```python
from build123d import *

# Parameters (mm, degrees)
SKETCH1_W                   = 31.9
SKETCH1_H                   = 17.8
SKETCH1_W_2                 = 22.5
SKETCH1_H_2                 = 11.8
BOSS_EXTRUDE1_DEPTH         = 8
BOSS_EXTRUDE2_DEPTH         = 16
SKETCH5_W                   = 14.05
SKETCH5_H                   = 12
SKETCH5_W_2                 = 15.95
SKETCH5_H_2                 = 8
BOSS_EXTRUDE3_DEPTH         = 3
CUT_EXTRUDE2_DEPTH          = 3
CUT_EXTRUDE3_DEPTH          = 43.272216091
BOSS_EXTRUDE4_START         = -8
BOSS_EXTRUDE4_DEPTH         = 8
CUT_EXTRUDE4_DEPTH          = 43.128612605
IZIM1_W                     = 73.483837375
IZIM1_H                     = 17.110844689
IZIM1_R                     = 4
Y_KSEKLIK_EKSTR_ZYON1_DEPTH = 30


with BuildPart() as part:
    # Sketch1 → Boss-Extrude1 (new body)
    with BuildSketch(Plane(origin=(0, 0, 0), x_dir=(1, 0, 0), z_dir=(0, 1, 0))):
        Rectangle(SKETCH1_W, SKETCH1_H)
        Rectangle(SKETCH1_W_2, SKETCH1_H_2, mode=Mode.SUBTRACT)
    extrude(amount=BOSS_EXTRUDE1_DEPTH)

    # Sketch3 → Boss-Extrude2 (add)
    with BuildSketch(Plane.XZ):
        with BuildLine():
            ThreePointArc((28.95, -7.4), (23.95, -12.4), (18.95, -7.4))
            Line((18.95, -7.4), (18.95, 18.9))
            Line((18.95, 18.9), (15.95, 18.9))
            Line((15.95, 18.9), (15.95, -8.9))
            ThreePointArc((15.95, -8.9), (24.70323224, -15.504482784), (32.089410298, -7.4))
            Line((32.089410298, -7.4), (32.089410298, 18.9))
            Line((32.089410298, 18.9), (28.95, 18.9))
            Line((28.95, 18.9), (28.95, -7.4))
        make_face()
    extrude(amount=-BOSS_EXTRUDE2_DEPTH)

    # Sketch5 → Boss-Extrude3 (add)
    with BuildSketch(Plane(origin=(0, 0, -8.9), x_dir=(-1, 0, 0), z_dir=(0, 0, -1))):
        with Locations((-7.025, 14)):
            Rectangle(SKETCH5_W, SKETCH5_H)
        with Locations((7.975, 14)):
            Rectangle(SKETCH5_W_2, SKETCH5_H)
        with Locations((7.975, 4)):
            Rectangle(SKETCH5_W_2, SKETCH5_H_2)
        with Locations((-7.025, 4)):
            Rectangle(SKETCH5_W, SKETCH5_H_2)
    extrude(amount=BOSS_EXTRUDE3_DEPTH)

    # Sketch6 → Cut-Extrude2 (cut)
    with BuildSketch(Plane.XY.offset(-8.9)):
        with BuildLine():
            Line((-11.95, 18), (10.05, 18))
            ThreePointArc((10.05, 18), (11.05, 17), (10.05, 16))
            Line((10.05, 16), (-11.95, 16))
            ThreePointArc((-11.95, 16), (-12.95, 17), (-11.95, 18))
        make_face()
        with BuildLine():
            Line((-11.95, 13), (10.05, 13))
            ThreePointArc((10.05, 13), (11.05, 12), (10.05, 11))
            Line((10.05, 11), (-11.95, 11))
            ThreePointArc((-11.95, 11), (-12.95, 12), (-11.95, 13))
        make_face()
    extrude(amount=-CUT_EXTRUDE2_DEPTH, mode=Mode.SUBTRACT)

    # Sketch7 → Cut-Extrude3 (cut, through all)
    with BuildSketch(Plane.XZ):
        with BuildLine():
            Line((-15.95, -0.393894215), (-15.95, 0.393894215))
            Line((-15.95, 0.393894215), (-14.56915578, 0.393894215))
            ThreePointArc((-14.56915578, 0.393894215), (-12.65, 0), (-14.56915578, -0.393894215))
            Line((-14.56915578, -0.393894215), (-15.95, -0.393894215))
        make_face()
    cut_extrude3 = extrude(amount=-CUT_EXTRUDE3_DEPTH, mode=Mode.SUBTRACT)

    # Mirror1: Cut-Extrude3 across plane
    add(cut_extrude3.mirror(Plane(origin=(0, 0, 0), x_dir=(0, 0, 1), z_dir=(1, 0, 0))), mode=Mode.SUBTRACT)

    # Sketch8 → Boss-Extrude4 (add)
    with BuildSketch(Plane.XZ.offset(BOSS_EXTRUDE4_START)):
        with BuildLine():
            Line((14.05, -11.9), (14.05, -8.9))
            Line((14.05, -8.9), (15.95, -8.9))
            ThreePointArc((15.95, -8.9), (16.408162032, -10.461156655), (17.167670017, -11.9))
            Line((17.167670017, -11.9), (14.05, -11.9))
        make_face()
    extrude(amount=BOSS_EXTRUDE4_DEPTH)

    # Sketch9 → Cut-Extrude4 (cut, through all)
    with BuildSketch(Plane.ZY.offset(-15.95)):
        with BuildLine():
            ThreePointArc((13.9, 15), (10.9, 12), (13.9, 9))
            Line((13.9, 9), (13.9, 15))
        make_face()
        with BuildLine():
            Line((13.9, 15), (13.9, 9))
            ThreePointArc((13.9, 9), (16.021320344, 9.878679656), (16.9, 12))
            ThreePointArc((16.9, 12), (16.021320344, 14.121320344), (13.9, 15))
        make_face()
    extrude(amount=-CUT_EXTRUDE4_DEPTH, mode=Mode.SUBTRACT)

    # Çizim1 → Yükseklik-Ekstrüzyon1 (add, symmetric)
    with BuildSketch(Plane.XZ):
        with Locations((20.791918688, -18.853722133)):
            Rectangle(IZIM1_W, IZIM1_H)
        with Locations(Location((48.791918688, -18.853722132, 0), (0, 0, 90))):
            Circle(IZIM1_R, mode=Mode.SUBTRACT)
        with Locations(Location((-7.208081312, -18.853722132, 0), (0, 0, 90))):
            Circle(IZIM1_R, mode=Mode.SUBTRACT)
    extrude(amount=Y_KSEKLIK_EKSTR_ZYON1_DEPTH, both=True)


solid = part.part
```
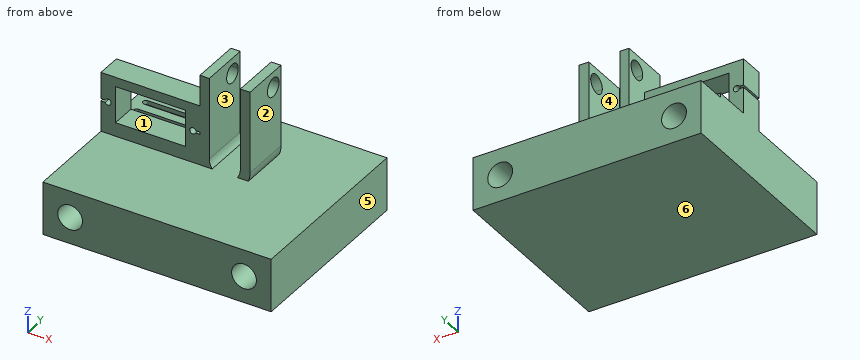
Geometry check sheet. Reference: the model listing, model coordinates, mm. Face numbers are marked on the shaded views. A direction names the side the tool comes from. Give positions to 0.01 mm unless a question says otherwise; leave off trailing zeros. Write each loop counter-clockwise with the first axis right and the second up, starting at its lowest first coordinate (ties: lowest second). Pieces come first, ordered by that corner, then holes. Notation, with made-up numbers: (24.5, -24) -> (59.5, -24) arc R24 ccw to (59.5, -4) -> close; hole circle Ø8 at (48.25, 47). An arc over 180 degrees is marked (long way). One line per question, with ' | ' between items.
Item 1: Draft check along X on the marked faces 4, 5 and 6. Enter one of: released by +X, released by -X, zero draft, split by the parting line, or undercut.
Determined:
face 4: undercut | face 5: released by +X | face 6: zero draft
Item 2: Sectioned sample at B-B, the plane z = -2. Record the boundary of the cut face in (x, y).
Determined:
outline: (-15.95, 0) -> (-11.25, 0) -> (-11.25, 8) -> (-15.95, 8) -> close; (11.25, 0) -> (18.95, 0) -> (18.95, 16) -> (15.95, 16) -> (15.95, 8) -> (11.25, 8) -> close; (28.95, 0) -> (32.09, 0) -> (32.09, 16) -> (28.95, 16) -> close
Item 3: Depth check by flat-ended pin: pin 1 (0.7 mm diameter, centred on x = -8, z = -9.5, fed in from +Y); pin 2 (1.2 mm diameter, centred on x = 19, z = 2.5, fed in from +Y); pin 3 (1.1 mm diameter, centred on y = 13, z = -9.5, fed in from +X). Enter the tip coordinate at first touch or a pass-through.
Determined:
pin 1: y = 20 | pin 2: y = 16 | pin 3: x = 31.94
Item 4: Sectioned sample at A-A, the plane z = 7.5. Record the boundary of the cut face in (x, y), plus the area to 3 significant figures.
Determined:
outline: (-15.95, 0) -> (18.95, 0) -> (18.95, 16) -> (15.95, 16) -> (15.95, 8) -> (-15.95, 8) -> close; (28.95, 0) -> (32.09, 0) -> (32.09, 16) -> (28.95, 16) -> close | area: 353 mm^2
Item 5: Sectioned sample at D-D, the plane y = -4. Record the boundary of the cut face in (x, z).
Determined:
outline: (-15.95, -27.41) -> (57.53, -27.41) -> (57.53, -10.3) -> (-15.95, -10.3) -> close; hole circle Ø8 at (-7.21, -18.85); hole circle Ø8 at (48.79, -18.85)
Item 6: Scan lines: line 1 along X through (y, z) = (4, 0); line 2 along X through (y, z) = (12, -9); line 3 along Z through (x, y) = (0, -21.5). Record each from-to range of solid material in increasing order.
Determined:
line 1: -12.65 to -11.25, 11.25 to 12.65, 15.95 to 18.95, 28.95 to 32.09 | line 2: -15.95 to -12.95, 11.05 to 14.05, 15.97 to 19.21, 28.69 to 31.93 | line 3: -27.41 to -10.3
Item 7: Access from +Z, -Z, +X, -X, +Y, -Y to the whole of each face (thin tool, end or side, straight path). Record for the marked faces 1, 2 and 3.
Determined:
face 1: +Y, -Y | face 2: +Z, +X, +Y, -Y | face 3: +Z, +Y, -Y
Item 8: Sectioned sample at C-C, the plane x = -9. Record the boundary of the cut face in (y, z), plus the area to 3 significant figures.
Determined:
outline: (-30, -27.41) -> (30, -27.41) -> (30, -22.43) -> (-30, -22.43) -> close; (-30, -15.28) -> (30, -15.28) -> (30, -10.3) -> (20, -10.3) -> (20, -8.9) -> (18, -8.9) -> (18, -10.3) -> (16, -10.3) -> (16, -8.9) -> (13, -8.9) -> (13, -10.3) -> (11, -10.3) -> (11, -8.9) -> (8, -8.9) -> (8, -5.9) -> (0, -5.9) -> (0, -10.3) -> (-30, -10.3) -> close; (0, 5.9) -> (8, 5.9) -> (8, 8.9) -> (0, 8.9) -> close | area: 668 mm^2
